from build123d import *

# Parameters (mm, degrees)
BOSS_EXTRUDE1_DEPTH             = 419.1
SKETCH2_W                       = 406.4
SKETCH2_H                       = 406.4
CUT_EXTRUDE1_DEPTH              = 406.4
BOSS_EXTRUDE2_START             = -505.46
BOSS_EXTRUDE2_DEPTH             = 1010.92
CUT_EXTRUDE2_DEPTH              = 453.007941176
CUT_EXTRUDE2_DEPTH_BACK         = 559.912058824
BOSS_EXTRUDE3_REACH             = 409.409
BOSS_EXTRUDE3_DIRECTION_2_REACH = 605.511


with BuildPart() as part:
    # Sketch1 → Boss-Extrude1 (new body)
    with BuildSketch(Plane(origin=(0, 0, 0), x_dir=(1, 0, 0), z_dir=(0, 1, 0))):
        Polygon((-111.498529412, 263.002058824), (-111.498529412, 558.912058824), (307.601470588, 558.912058824), (307.601470588, 263.002058824), (603.511470588, 263.002058824), (603.511470588, -156.097941176), (307.601470588, -156.097941176), (307.601470588, -452.007941176), (-111.498529412, -452.007941176), (-111.498529412, -156.097941176), (-407.408529412, -156.097941176), (-407.408529412, 263.002058824), align=None)
    extrude(amount=BOSS_EXTRUDE1_DEPTH)

    # Sketch2 → Cut-Extrude1 (cut)
    with BuildSketch(Plane.ZY.offset(407.408529412)):
        with Locations((-53.452058824, 209.55)):
            Rectangle(SKETCH2_W, SKETCH2_H)
    cut_extrude1 = extrude(amount=-CUT_EXTRUDE1_DEPTH, mode=Mode.SUBTRACT)

    # Mirror1: Cut-Extrude1 across plane
    add(cut_extrude1.mirror(Plane.ZY.offset(-98.051470588)), mode=Mode.SUBTRACT)

    # Sketch3 → Boss-Extrude2 (add)
    with BuildSketch(Plane.ZY.offset(-98.051470588).offset(BOSS_EXTRUDE2_START)):
        Polygon((-205.790064307, 419.1), (98.88594666, 419.1), (155.185867753, 620.042461281), (106.481982696, 706.660847592), (0, 744.864396526), (-106.904117647, 744.864396526), (-213.386100343, 706.660847592), (-262.0899854, 620.042461281), align=None)
    extrude(amount=BOSS_EXTRUDE2_DEPTH)

    # Sketch4 → Cut-Extrude2 (cut, two sides)
    with BuildSketch(Plane.XY) as cut_extrude2_sk:
        Polygon((-305.808529412, 425.454129149), (-394.708529412, 577.854129149), (-394.708529412, 796.580225866), (590.811470588, 796.580225866), (590.811470588, 573.314003685), (501.911470588, 420.914003685), (647.189097077, 420.914003685), (647.189097077, 885.635632277), (-516.891145843, 876.882773083), (-501.7416469, 425.454129149), align=None)
    extrude(amount=CUT_EXTRUDE2_DEPTH, mode=Mode.SUBTRACT)
    extrude(cut_extrude2_sk.sketch, amount=-CUT_EXTRUDE2_DEPTH_BACK, mode=Mode.SUBTRACT)

    # Boss-Extrude3: up to this face of the body (flat: up to its plane)
    boss_extrude3_end = Plane(part.part.faces().sort_by_distance((-111.498529412, 209.55, 304.052941176))[0])
    # Sketch5 → Boss-Extrude3 (add, up to the picked face)
    with BuildSketch(Plane(origin=(0, 0, 0), x_dir=(0, 0, -1), z_dir=(1, 0, 0)), mode=Mode.PRIVATE) as boss_extrude3_sk1:
        Polygon((-449.181000693, 419.206207419), (-542.705165158, 559.069271968), (-471.821113531, 655.706983405), (-471.821113531, 732.000172587), (-466.55643227, 739.177622759), (510.328311202, 739.177622759), (517.505761373, 732.000172587), (517.505761373, 655.706983405), (576.040352368, 576.087761543), (512.785450653, 419.206207419), align=None)
    boss_extrude3_tool1 = split(extrude(boss_extrude3_sk1.sketch, amount=-BOSS_EXTRUDE3_REACH, mode=Mode.PRIVATE), bisect_by=boss_extrude3_end, keep=Keep.BOTH, mode=Mode.PRIVATE)
    add(boss_extrude3_tool1.solids().sort_by_distance((0, 578.35257, -22.327279))[0])

    # Boss-Extrude3 direction 2: up to this face of the body (flat: up to its plane)
    boss_extrude3_direction_2_end = Plane(part.part.faces().sort_by_distance((307.601470588, 209.55, 304.052941176))[0])
    # Sketch5 → Boss-Extrude3 direction 2 (add, up to the picked face)
    with BuildSketch(Plane(origin=(0, 0, 0), x_dir=(0, 0, -1), z_dir=(1, 0, 0)), mode=Mode.PRIVATE) as boss_extrude3_direction_2_sk1:
        Polygon((-449.181000693, 419.206207419), (-542.705165158, 559.069271968), (-471.821113531, 655.706983405), (-471.821113531, 732.000172587), (-466.55643227, 739.177622759), (510.328311202, 739.177622759), (517.505761373, 732.000172587), (517.505761373, 655.706983405), (576.040352368, 576.087761543), (512.785450653, 419.206207419), align=None)
    boss_extrude3_direction_2_tool1 = split(extrude(boss_extrude3_direction_2_sk1.sketch, amount=BOSS_EXTRUDE3_DIRECTION_2_REACH, mode=Mode.PRIVATE), bisect_by=boss_extrude3_direction_2_end, keep=Keep.BOTH, mode=Mode.PRIVATE)
    add(boss_extrude3_direction_2_tool1.solids().sort_by_distance((0, 578.35257, -22.327279))[0])


solid = part.part
Build history of the part. All positions in model axes, mm. A direction names the side the tool comes from. Round coordinates to 2 decimals unless told otherwise and drop trailing zeros. Loops run counter-clockwise (first coordinate to the right, second up) from the corner with the lowest first, then second, coordinate; pieces in that order, holes last. Notation, with made-up numbers: (25.5, -19) -> (29.5, -19) arc R24 cw to (29.5, 16) -> close; hole circle Ø3 at (81.25, -18.75). An arc over 180 degrees is marked (long way). Answer in a Markdown table with one row per item.
Item 1: Pin check, flat tips, straight feed: pin 1 (4 mm diameter, centred on x = 54.5, z = -436.5, fed in from +Y); pin 2 (1.5 mm diameter, centred on x = 86, y = 536.5, fed in from +Z) (3 decimals); pin 3 (3 mm diameter, centred on x = 275.5, y = 541, fed in from -Z); pin 4 (3 mm diameter, centred on x = 279, z = -132.5, fed in from -Y). Stop position of each tip, or through.
Answers below:
| item | result |
|---|---|
| pin 1 | stops at y = 739.18 |
| pin 2 | stops at z = 528.115 |
| pin 3 | stops at z = -562.5 |
| pin 4 | stops at y = 0 |
Item 2: Drill centre lines: L1, parallel to Z at x = -67.5, y = 202.5; L2, parallel to Z at x = -252.5, y = 186; L3, parallel to Y at x = 269.5, z = -2. Where is each one in solid material? Low to high. Write a range as [from, to].
Answers below:
| item | result |
|---|---|
| L1 | z = [-558.91, -256.65], [149.75, 452.01] |
| L2 | z = [-263, -256.65], [149.75, 156.1] |
| L3 | y = [0, 6.35], [412.75, 744.86] |
Item 3: Which spindle directions (+Z, -Z, +X, -X, +Y, -Y) get a long thin tool onto all of the face, cutting with end or side? Do faces 4 (the flat face through (95.118, 498.745, -544.856)), 5 (the flat face through (95, 693, 471.821)), 6 (the flat face through (-207, 412.75, -56)). Say none if no direction does.
Answers below:
| item | result |
|---|---|
| face 4 | -Z, +X, -X |
| face 5 | +Z, +X, -X, +Y |
| face 6 | -X |
Item 4: Saw through at A-A (z = 372). Write the cut outline in (x, y).
Answers below:
| item | result |
|---|---|
| outline | (-111.5, 0) -> (307.6, 0) -> (307.6, 419.1) -> (-111.5, 419.1) -> close; (-111.5, 419.21) -> (307.6, 419.21) -> (307.6, 739.18) -> (-111.5, 739.18) -> close |
Item 5: Saw through at C-C (x = 536). Write the cut outline in (y, z).
Answers below:
| item | result |
|---|---|
| outline | (0, -263) -> (419.1, -263) -> (419.1, -205.79) -> (420.91, -206.3) -> (420.91, 99.39) -> (419.1, 98.89) -> (419.1, 156.1) -> (0, 156.1) -> close; (479.35, -222.67) -> (620.04, -262.09) -> (706.66, -213.39) -> (744.86, -106.9) -> (744.86, 0) -> (706.66, 106.48) -> (620.04, 155.19) -> (479.35, 115.77) -> close; hole (6.35, -256.65) -> (412.75, -256.65) -> (412.75, 149.75) -> (6.35, 149.75) -> close |
Item 6: Mould opens along Y. For faces 1 (the flat face through (105, 743, -112.1)), 2 (the flat face through (95, 207, -558.912)), 3 (the flat face through (-207, 207, -256.652)) say: +Y half, -Y half, draft (parallel to the pull), parting line (faces both ways), or undercut.
Answers below:
| item | result |
|---|---|
| face 1 | +Y half |
| face 2 | draft |
| face 3 | undercut |
Item 7: Saw through at D-D (z = -79). Write the cut outline in (x, y).
Answers below:
| item | result |
|---|---|
| outline | (-407.41, 0) -> (603.51, 0) -> (603.51, 6.35) -> (197.11, 6.35) -> (197.11, 412.75) -> (603.51, 412.75) -> (603.51, 420.91) -> (501.91, 420.91) -> (590.81, 573.31) -> (590.81, 744.86) -> (-394.71, 744.86) -> (-394.71, 577.85) -> (-305.81, 425.45) -> (-407.41, 425.45) -> (-407.41, 412.75) -> (-1.01, 412.75) -> (-1.01, 6.35) -> (-407.41, 6.35) -> close |
Item 8: Saw through at B-B (x = -191). Write the cut outline in (y, z), and give its area (3 significant figures).
Answers below:
| item | result |
|---|---|
| outline | (0, -263) -> (419.1, -263) -> (419.1, -205.79) -> (620.04, -262.09) -> (706.66, -213.39) -> (744.86, -106.9) -> (744.86, 0) -> (706.66, 106.48) -> (620.04, 155.19) -> (419.1, 98.89) -> (419.1, 156.1) -> (0, 156.1) -> close; hole (6.35, -256.65) -> (412.75, -256.65) -> (412.75, 149.75) -> (6.35, 149.75) -> close |
| area | 123,000 mm² |
